from build123d import *

# Parameters (mm, degrees)
SKETCH2_R          = 12.5
CUT_EXTRUDE1_DEPTH = 70
SKETCH5_R          = 4
CUT_EXTRUDE2_DEPTH = 27


with BuildPart() as part:
    # Sketch1 → Revolve1 (revolve)
    with BuildSketch(Plane(origin=(0, 0, 0), x_dir=(1, 0, 0), z_dir=(0, 1, 0)), mode=Mode.PRIVATE) as revolve1_sk:
        Polygon((0, 24.303944316), (40, 24.303944316), (40, 19.303944316), (25, 15.553944316), (25, 3.053944316), (40, -0.696055684), (40, -5.696055684), (25, -5.696055684), (25, -25.696055684), (0, -25.696055684), align=None)
    revolve(revolve1_sk.sketch.rotate(Axis((0, 0, -24.303944316), (0, 0, 1)), 180), axis=Axis((0, 0, -24.303944316), (0, 0, 1)))

    # Sketch2 → Cut-Extrude1 (cut)
    with BuildSketch(Plane.XY.offset(25.696055684)):
        Circle(SKETCH2_R)
    extrude(amount=-CUT_EXTRUDE1_DEPTH, mode=Mode.SUBTRACT)

    # Sketch5 → Cut-Extrude2 (cut)
    with BuildSketch(Plane(origin=(0, 25, 25.696055684), x_dir=(1, 0, 0), z_dir=(0, 1, 0))):
        with Locations(Location((0, 11.058273662, 0), (0, 0, 180))):
            Circle(SKETCH5_R)
    extrude(amount=-CUT_EXTRUDE2_DEPTH, mode=Mode.SUBTRACT)


solid = part.part
For this review, take the finished solid that the model builds, in its own axes (mm). A direction names the side the tool comes from. Round coordinates to 2 decimals unless told otherwise and drop trailing zeros. Write each loop counter-clockwise with the first axis right and the second up, starting at its lowest first coordinate (ties: lowest second). Pieces come first, ordered by that corner, then holes. Notation, with made-up numbers: (-37, 18) - (-3, 18) arc R8 cw to (-3, 27) - close; hole circle Ø6 at (9, 16.25). An arc over 180 degrees is marked (long way). Use a Markdown table: item, result.
Q1. We need section D-D (z = -1). Give the boundary of the cut face in (x, y).
Derived:
| item | result |
|---|---|
| outline | circle Ø66.43 at (0, 0); hole circle Ø25 at (0, 0) |
Q2. Wall thickness on line 1 along Y through (x, z) = (0, -5); line 2 along Y through (x, z) = (0, 1.5); line 3 along Z through (x, y) = (3, 18): over which ranges is each line inside the solid? List them lowest first.
Derived:
| item | result |
|---|---|
| line 1 | y = -25 to -12.5, 12.5 to 25 |
| line 2 | y = -40 to -12.5, 12.5 to 40 |
| line 3 | z = -24.3 to 11.99, 17.28 to 25.7 |
Q3. The part is to be moulded in two halves that separate along Z. For faces 4 (the cylindrical face through (39.96, -1.76, 3.23)), 5 (the flat face through (-9, -9, -24.304)), 6 (the flat face through (-17.22, -18.34, 5.696)), 7 (the conical face through (5.577, 25.117, -15.736)), say which applies: pulls with the +Z half, pulls with the -Z half, needs draft (parallel to the pull), parting line crosses it, or undercut.
Derived:
| item | result |
|---|---|
| face 4 | needs draft |
| face 5 | pulls with the -Z half |
| face 6 | pulls with the +Z half |
| face 7 | undercut |
Q4. Machinability: for faces 1 (the cylindrical face through (-23.846, -7.509, 15.836)), 2 (the cylindrical face through (0.867, 18.514, 10.733)), 3 (the cylindrical face through (-23.846, -7.509, -9.216)), which of the approach directions +Z, -Z, +X, -X, +Y, -Y give a long, thin tool a straight path to every point of the face, cutting with its end or side? Answer none if there is none.
Derived:
| item | result |
|---|---|
| face 1 | +Z |
| face 2 | +Y |
| face 3 | none |
Q5. Clearance check with flat-ended pins moving along their axes: pin 1 (5 mm diameter, centred on x = 0, z = 14.64, fed in from +Y); pin 2 (5 mm diameter, centred on x = 7, z = -19, fed in from +Y); pin 3 (5 mm diameter, centred on x = 6, z = 8, fed in from -Y). State where each tip first meets the part, or that it passes through.
Derived:
| item | result |
|---|---|
| pin 1 | stops at y = -12.25 |
| pin 2 | stops at y = 39.74 |
| pin 3 | stops at y = -39.68 |
Q6. We need section B-B (x = 0). Give the boundary of the cut face in (y, z), plus the area to 3 significant figures.
Derived:
| item | result |
|---|---|
| outline | (-40, -24.3) - (-12.5, -24.3) - (-12.5, 25.7) - (-25, 25.7) - (-25, 5.7) - (-40, 5.7) - (-40, 0.7) - (-25, -3.05) - (-25, -15.55) - (-40, -19.3) - close; (12.5, -24.3) - (40, -24.3) - (40, -19.3) - (25, -15.55) - (25, -3.05) - (40, 0.7) - (40, 5.7) - (25, 5.7) - (25, 10.64) - (12.5, 10.64) - close; (12.5, 18.64) - (25, 18.64) - (25, 25.7) - (12.5, 25.7) - close |
| area | 1,560 mm2 |
Q7. We need section A-A (y = 0). Give the boundary of the cut face in (x, z), plus the area to 3 significant figures.
Derived:
| item | result |
|---|---|
| outline | (-40, -24.3) - (-12.5, -24.3) - (-12.5, 25.7) - (-25, 25.7) - (-25, 5.7) - (-40, 5.7) - (-40, 0.7) - (-25, -3.05) - (-25, -15.55) - (-40, -19.3) - close; (12.5, -24.3) - (40, -24.3) - (40, -19.3) - (25, -15.55) - (25, -3.05) - (40, 0.7) - (40, 5.7) - (25, 5.7) - (25, 25.7) - (12.5, 25.7) - close |
| area | 1,660 mm2 |
Q8. We need section C-C (z = -14). Give the boundary of the cut face in (x, y), plus the area to 3 significant figures.
Derived:
| item | result |
|---|---|
| outline | circle Ø50 at (0, 0); hole circle Ø25 at (0, 0) |
| area | 1,470 mm2 |
